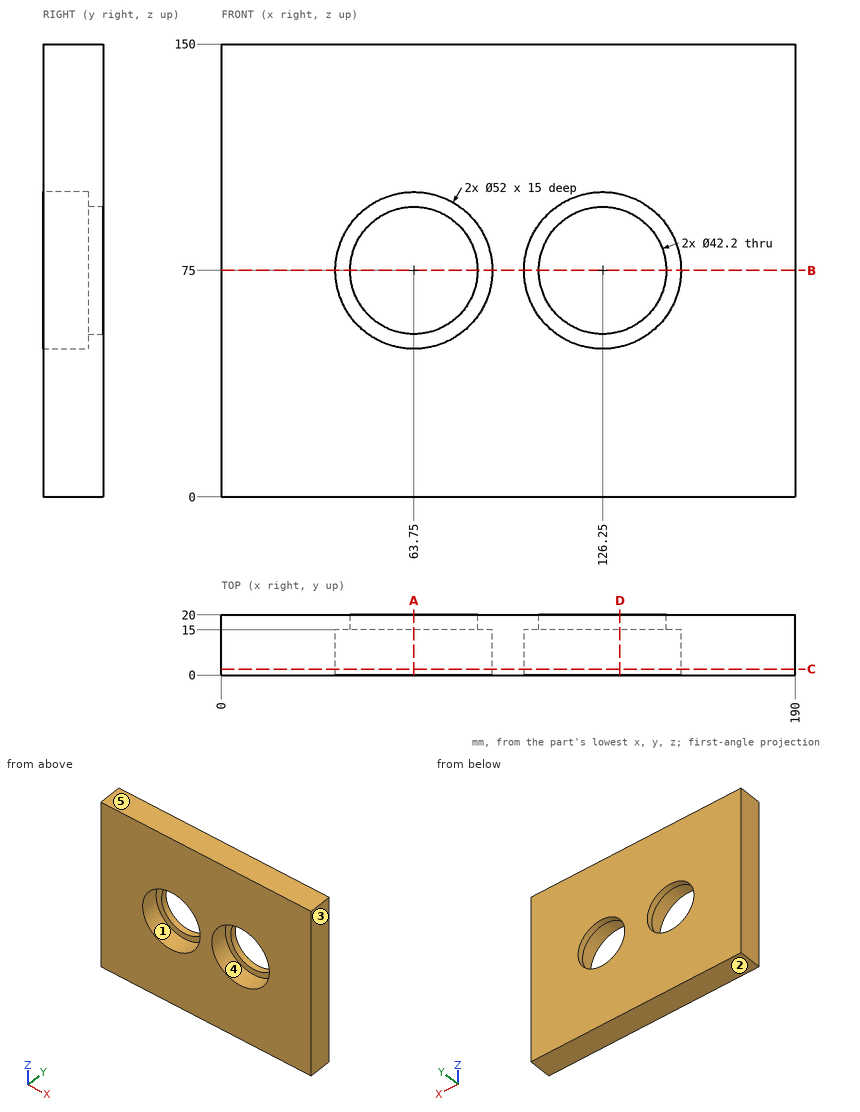
Study the drawing (mm; zero at the part's minimum x, y, z) and answer. A direction names the side the tool comes from. Give positions to 0.01 mm unless a question says otherwise; leave off trailing zeros. Write each loop counter-clockwise with the first axis right and the second up, starting at its lowest first coordinate (ties: lowest second). Pieces come first, ordered by that corner, then holes. Notation, with made-up numbers: (65, 51) -> (93, 51) arc R34 ccw to (93, 82) -> close; hole circle Ø8 at (53, 82.25). An arc over 180 degrees is marked (long way). Write item = value, one per line.
Q1. Section C-C on y = 2 is taken. Determine the outline of the cut face in (x, z).
Computed values:
outline = (0, 0) -> (190, 0) -> (190, 150) -> (0, 150) -> close; hole circle Ø52 at (63.75, 75); hole circle Ø52 at (126.25, 75)
Q2. Section B-B on z = 75 is taken. Determine the outline of the cut face in (x, y).
Computed values:
outline = (0, 0) -> (37.75, 0) -> (37.75, 15) -> (42.65, 15) -> (42.65, 20) -> (0, 20) -> close; (84.85, 15) -> (89.75, 15) -> (89.75, 0) -> (100.25, 0) -> (100.25, 15) -> (105.15, 15) -> (105.15, 20) -> (84.85, 20) -> close; (147.35, 15) -> (152.25, 15) -> (152.25, 0) -> (190, 0) -> (190, 20) -> (147.35, 20) -> close
Q3. For a pull along X with two mould halves and no side action, classify the marked faces 1, 2 and 3 as pulls with the +X half, pulls with the -X half, needs draft (parallel to the pull), parting line crosses it, or undercut.
Computed values:
face_1 = undercut
face_2 = needs draft
face_3 = pulls with the +X half
Q4. Section A-A on x = 63.75 is taken. Determine the outline of the cut face in (y, z).
Computed values:
outline = (0, 0) -> (20, 0) -> (20, 53.9) -> (15, 53.9) -> (15, 49) -> (0, 49) -> close; (0, 101) -> (15, 101) -> (15, 96.1) -> (20, 96.1) -> (20, 150) -> (0, 150) -> close
Q5. Consider line 1 along X through (y, z) = (4.75, 75); line 2 along X through (y, z) = (16.3, 75); line 3 along Y through (x, z) = (120, 50.5). Determine where each line is inside the solid, lowest interval first.
Computed values:
line_1 = 0 to 37.75, 89.75 to 100.25, 152.25 to 190
line_2 = 0 to 42.65, 84.85 to 105.15, 147.35 to 190
line_3 = 15 to 20
Q6. A tool of negligible diameter and unlimited length cuts with its end or side. For the marked faces 4 and 5, from which of +Z, -Z, +X, -X, +Y, -Y can it reach the whole face along a straight path? Write none if from no direction.
Computed values:
face_4 = -Y
face_5 = +Z, +X, -X, +Y, -Y
Q7. Section D-D on x = 132 is taken. Determine the outline of the cut face in (y, z), and give its area (3 significant figures).
Computed values:
outline = (0, 0) -> (20, 0) -> (20, 54.7) -> (15, 54.7) -> (15, 49.64) -> (0, 49.64) -> close; (0, 100.36) -> (15, 100.36) -> (15, 95.3) -> (20, 95.3) -> (20, 150) -> (0, 150) -> close
area = 2,040 mm^2
